Here's the drawing with two shaded views (mm, measured from the low corner). I have some questions. A direction names the side the tool comes from. Give positions to 0.01 mm unless a question says otherwise; leave off trailing zeros. Loops run counter-clockwise (first coordinate to the right, second up) from the corner with the lowest first, then second, coordinate; pieces in that order, holes last. Notation, with made-up numbers: M -10.75,13 L 35.25,13 A7 ccw 35.25,24 Z; hole C 74,17 d8. An arc over 180 degrees is marked long. Use CSV: the item, a comma, the result in double quotes.
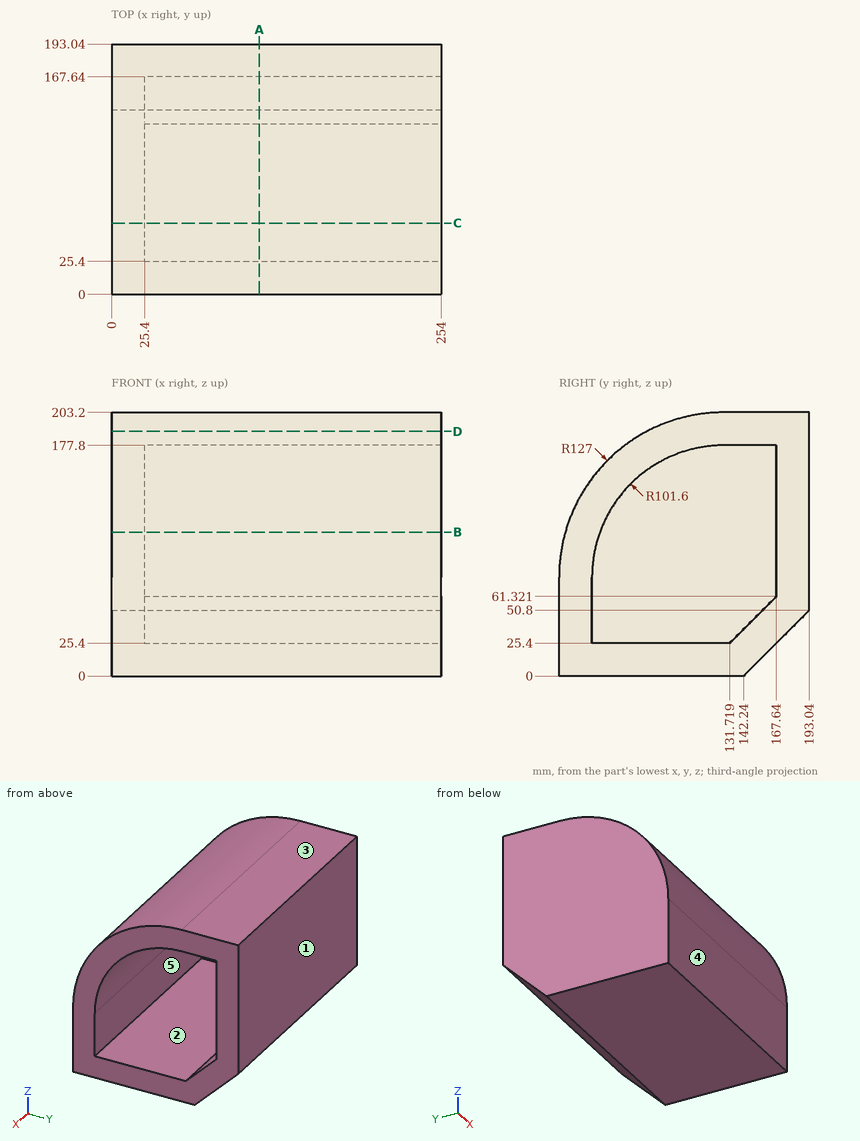
1. I'm going to push flat-ended pins straight in: pin 1 Ø8 at (y, z) = (152, 67) entering from +X; pin 2 Ø8 at (x, z) = (165, 106) entering from -Y; pin 3 Ø3 at (y, z) = (82.5, 122) entering from -X; pin 4 Ø12 at (x, y) = (190, 152) entering from -Z. Where does each tip first touch, or does it pass through?
Outcome:
pin 1,"x = 25.4"
pin 2,"y = 2.65"
pin 3,"x = 0"
pin 4,"z = 3.76"
2. I want a section at D-D, the plane z = 188.5. List the corners of the cut face in (x, y) for me.
Outcome:
outline,"M 0,67.69 L 254,67.69 L 254,193.04 L 0,193.04 Z"
3. Which directions (+Z, -Z, +X, -X, +Y, -Y) give clear straight access to the entire face, cutting with the end or side of a thin tool? Please do the marked faces 4 and 5.
Outcome:
face 4,"+Z, -Z, +X, -X, -Y"
face 5,"+X"
4. I want a section at A-A, the plane x = 114. List the corners of the cut face in (y, z) for me, then the cut area to 3 significant figures.
Outcome:
outline,"M 0,0 L 142.24,0 L 193.04,50.8 L 193.04,203.2 L 127,203.2 A127 ccw 0,76.2 Z; hole M 25.4,25.4 L 131.72,25.4 L 167.64,61.32 L 167.64,177.8 L 127,177.8 A101.6 ccw 25.4,76.2 Z"
area,"15,700 mm2"
5. Please list where these lines run through material, in increasing order: line 1 (X direction, y = 117.5, z = 83.5); line 2 (Z direction, x = 36.5, y = 160); line 3 (Z direction, x = 187.5, y = 40).
Outcome:
line 1,"0 to 25.4"
line 2,"17.76 to 53.68, 177.8 to 203.2"
line 3,"0 to 25.4, 128.67 to 168.72"
6. I want a section at C-C, the plane y = 55. List the corners of the cut face in (x, z) for me.
Outcome:
outline,"M 0,0 L 254,0 L 254,25.4 L 25.4,25.4 L 25.4,147.88 L 254,147.88 L 254,180.82 L 0,180.82 Z"
7. I want a section at B-B, the plane z = 111. List the corners of the cut face in (x, y) for me, then the cut area to 3 significant figures.
Outcome:
outline,"M 0,4.86 L 254,4.86 L 254,31.55 L 25.4,31.55 L 25.4,167.64 L 254,167.64 L 254,193.04 L 0,193.04 Z"
area,"16,700 mm2"
8. If we mould it in two halves opening along Z, with no side actions, what happens to the marked faces 1, 2 and 3? For each: +Z half, -Z half, draft (parallel to the pull), parting line (faces both ways), or undercut.
Outcome:
face 1,"draft"
face 2,"undercut"
face 3,"+Z half"
